For this review, use the dimensioned drawing (mm, ordinates from the lowest corner) and the shaded views. Give positions to 0.01 mm unless a question says otherwise; leave off trailing zeros. Loops run counter-clockwise (first coordinate to the right, second up) from the corner with the lowest first, then second, coordinate; pieces in that order, holes last. Notation, with made-up numbers: (0, 33.5) - (33, 33.5) arc R27 cw to (33, 72.5) - close; hole circle Ø8 at (55, 78.25). An arc over 180 degrees is marked (long way). Put each result on its own line as item: value.
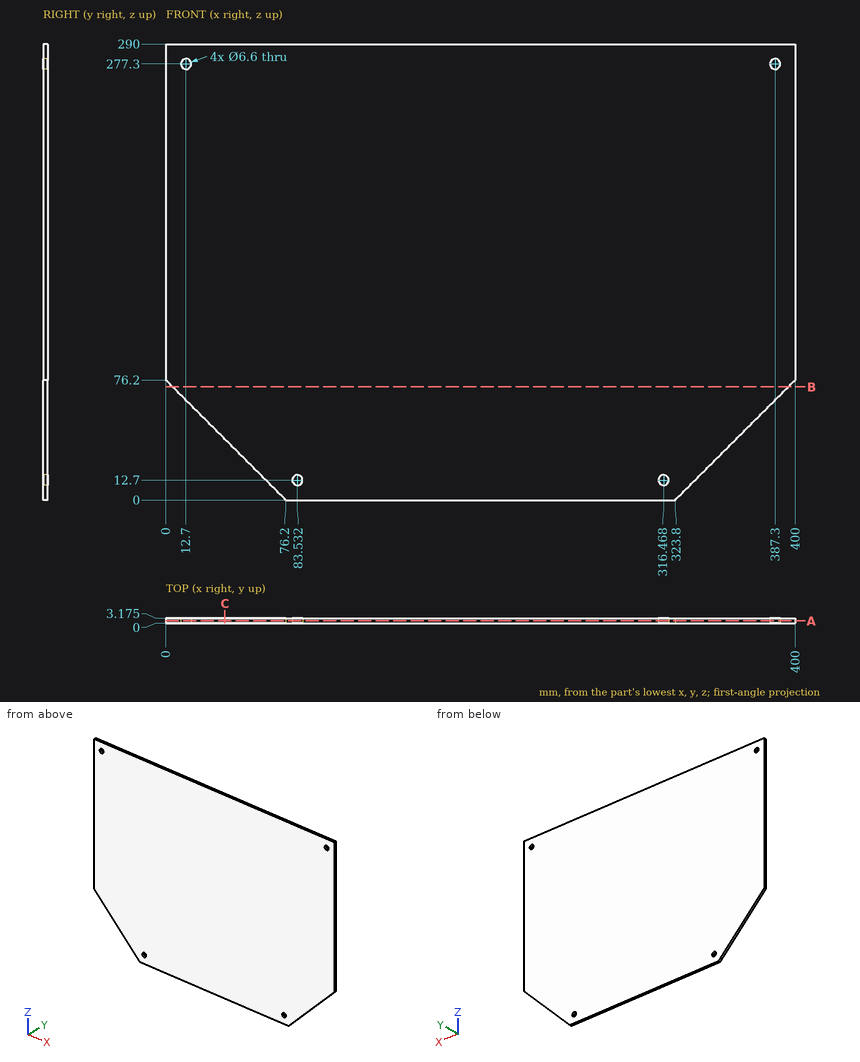
1) Take a section at C-C on x = 37.5. State the section outline as (y, z) points (1 decimal).
Geometry check:
outline: (0, 38.7) - (3.2, 38.7) - (3.2, 290) - (0, 290) - close
2) Wall thickness on line 1 (X direction, y = 1.75, z = 277.3); line 2 (X direction, y = 2.5, z = 12.7); line 3 (Z direction, x = 83, y = 1.95): over which ranges is each line inside the solid? List them lowest first.
Geometry check:
line 1: x = 0 to 9.4, 16 to 384, 390.6 to 400
line 2: x = 63.5 to 80.23, 86.83 to 313.17, 319.77 to 336.5
line 3: z = 0 to 9.44, 15.96 to 290
3) Insertion check: pin 1 Ø4 at (x, z) = (387.3, 277.3) entering from -Y. The pin has a flat end and moves straight along its axis. Give the tip position at first contact, or say it passes through.
Geometry check:
pin 1: passes through
4) Take a section at B-B on z = 72. State the section outline as (x, y) points (1 decimal).
Geometry check:
outline: (4.2, 0) - (395.8, 0) - (395.8, 3.2) - (4.2, 3.2) - close
5) Take a section at A-A on y = 1.4. State the section outline as (x, z) points, and give its area (3 significant figures).
Geometry check:
outline: (0, 76.2) - (76.2, 0) - (323.8, 0) - (400, 76.2) - (400, 290) - (0, 290) - close; hole circle Ø6.6 at (12.7, 277.3); hole circle Ø6.6 at (83.53, 12.7); hole circle Ø6.6 at (316.47, 12.7); hole circle Ø6.6 at (387.3, 277.3)
area: 110,000 mm²
